from build123d import *

# Parameters (mm, degrees)
SKETCH1_R           = 4.5
BOSS_EXTRUDE1_DEPTH = 8
SKETCH2_R           = 4
BOSS_EXTRUDE2_DEPTH = 3
SKETCH3_R           = 2
CUT_EXTRUDE1_DEPTH  = 5
BOSS_EXTRUDE3_DEPTH = 8
SKETCH5_W           = 7
SKETCH5_H           = 20
BOSS_EXTRUDE4_DEPTH = 12
FILLET1_START       = -13.395559342
FILLET1_DEPTH       = 7
FILLET1_2_DEPTH     = 7
SKETCH6_W           = 7
SKETCH6_H           = 8
CUT_EXTRUDE2_DEPTH  = 8
FILLET2_R           = 3
SKETCH7_R           = 1.75
CUT_EXTRUDE3_DEPTH  = 57.724097483


with BuildPart() as part:
    # Sketch1 → Boss-Extrude1 (new body)
    with BuildSketch(Plane(origin=(0, 0, 0), x_dir=(1, 0, 0), z_dir=(0, 1, 0))):
        with BuildLine():
            Line((0, 6), (11, 6))
            Line((11, 6), (11, -6))
            Line((11, -6), (0, -6))
            ThreePointArc((0, -6), (-6, 0), (0, 6))
        make_face()
        with Locations(Location((0, 0, 0), (0, 0, 270))):
            Circle(SKETCH1_R, mode=Mode.SUBTRACT)
    extrude(amount=BOSS_EXTRUDE1_DEPTH)

    # Sketch2 → Boss-Extrude2 (add)
    with BuildSketch(Plane(origin=(11, 0, 0), x_dir=(0, 0, -1), z_dir=(1, 0, 0))):
        with Locations(Location((0, 4, 0), (0, 0, 270))):
            Circle(SKETCH2_R)
    extrude(amount=BOSS_EXTRUDE2_DEPTH)

    # Sketch3 → Cut-Extrude1 (cut)
    with BuildSketch(Plane(origin=(14, 0, 0), x_dir=(0, 0, -1), z_dir=(1, 0, 0))):
        with Locations((0, 4)):
            Circle(SKETCH3_R)
    extrude(amount=-CUT_EXTRUDE1_DEPTH, mode=Mode.SUBTRACT)

    # Sketch4 → Boss-Extrude3 (add)
    with BuildSketch(Plane(origin=(0, 0, 0), x_dir=(1, 0, 0), z_dir=(0, 1, 0))):
        Polygon((0, -6), (0, -9.124355653), (-13.395559342, -32.326145029), (-13.395559342, -39.201789376), (-6.395559342, -39.201789376), (-6.395559342, -34.201789376), (7, -11), (7, -6), align=None)
    extrude(amount=BOSS_EXTRUDE3_DEPTH)

    # Sketch5 → Boss-Extrude4 (add)
    with BuildSketch(Plane.XY.offset(39.201789376)):
        with Locations((-9.895559342, 4)):
            Rectangle(SKETCH5_W, SKETCH5_H)
    extrude(amount=BOSS_EXTRUDE4_DEPTH)

    # Fillet1: read off the stored shape, not the designer's step
    # Fillet1 outline → Fillet1 (cut)
    with BuildSketch(Plane.YZ.offset(FILLET1_START)):
        with BuildLine():
            Line((-6, 39.201789376), (-3, 39.201789376))
            ThreePointArc((-3, 39.201789376), (-5.121320344, 40.080469032), (-6, 42.201789376))
            Line((-6, 42.201789376), (-6, 39.201789376))
        make_face()
        with BuildLine():
            ThreePointArc((14, 42.201789376), (13.121320344, 40.080469032), (11, 39.201789376))
            Line((11, 39.201789376), (14, 39.201789376))
            Line((14, 39.201789376), (14, 42.201789376))
        make_face()
    extrude(amount=FILLET1_DEPTH, mode=Mode.SUBTRACT)

    # Fillet1 2 outline → Fillet1 2 (add)
    with BuildSketch(Plane.YZ.offset(FILLET1_START)):
        with BuildLine():
            ThreePointArc((-3, 39.201789376), (-0.878679657, 38.32310972), (0, 36.201789376))
            Line((0, 36.201789376), (0, 39.201789376))
            Line((0, 39.201789376), (-3, 39.201789376))
        make_face()
        with BuildLine():
            ThreePointArc((8, 36.201789376), (8.878679656, 38.32310972), (11, 39.201789376))
            Line((11, 39.201789376), (8, 39.201789376))
            Line((8, 39.201789376), (8, 36.201789376))
        make_face()
    extrude(amount=FILLET1_2_DEPTH)

    # Sketch6 → Cut-Extrude2 (cut)
    with BuildSketch(Plane.XY.offset(51.201789376)):
        with Locations((-9.895559342, 4)):
            Rectangle(SKETCH6_W, SKETCH6_H)
    extrude(amount=-CUT_EXTRUDE2_DEPTH, mode=Mode.SUBTRACT)

    # Fillet2
    fillet2_edges = [part.edges().sort_by_distance(p)[0] for p in [
        (-6.395559342, -3, 51.201789376),
        (-13.395559342, 11, 51.201789376),
        (-6.395559342, 11, 51.201789376),
        (-13.395559342, -3, 51.201789376),
    ]]
    fillet(fillet2_edges, radius=FILLET2_R)

    # Sketch7 → Cut-Extrude3 (cut, through all)
    with BuildSketch(Plane(origin=(0, 14, 0), x_dir=(1, 0, 0), z_dir=(0, 1, 0))):
        with Locations(Location((-9.895559342, -47.201789376, 0), (0, 0, 180))):
            Circle(SKETCH7_R)
    extrude(amount=-CUT_EXTRUDE3_DEPTH, mode=Mode.SUBTRACT)


solid = part.part
Read the model definition and answer for the solid it produces. Units are mm, in the model's axes. A direction names the side the tool comes from. Give positions to 0.01 mm unless a question says otherwise; leave off trailing zeros. Loops run counter-clockwise (first coordinate to the right, second up) from the corner with the lowest first, then second, coordinate; pieces in that order, holes last. Notation, with made-up numbers: (76, 46) -> (94, 46) arc R27 ccw to (94, 76) -> close; hole circle Ø9 at (-27.5, 52.5). An arc over 180 degrees is marked (long way). Use a Markdown table: item, result.
Q1. Section B-B, the plane x = 9.75 is taken. Determine the outline of the cut face in (y, z).
Solved:
| item | result |
|---|---|
| outline | (0, -6) -> (8, -6) -> (8, 6) -> (0, 6) -> close; hole circle Ø4 at (4, 0) |
Q2. Find the intervals of material crossed by line 1 along Z through (x, y) = (-1, 2.5); line 2 along Y through (x, z) = (-6.5, 45); line 3 along Y through (x, z) = (-4.5, 1.5), in increasing order.
Solved:
| item | result |
|---|---|
| line 1 | z = -5.92 to -4.39, 4.39 to 5.92, 10.86 to 24.86 |
| line 2 | y = -6 to 0, 8 to 14 |
| line 3 | y = 0 to 8 |
Q3. A tool of negligible diameter and unlimited length cuts with its end or side. For faces 5 (the face through (-6.396, 4, 41)), 6 (the face through (-12, 8, 46)), 7 (the face through (11, 3.9, -4.4)), 8 (the face through (0, 4, 8)), from which of +Z, -Z, +X, -X, +Y, -Y can it reach the whole face along a straight path? Write none if from no direction.
Solved:
| item | result |
|---|---|
| face 5 | +Z, +X, +Y, -Y |
| face 6 | +Z, +X, -X |
| face 7 | -Z, +X |
| face 8 | -X, +Y, -Y |
Q4. Section A-A, the plane y = 4 is taken. Determine the outline of the cut face in (x, z).
Solved:
| item | result |
|---|---|
| outline | (-13.4, 32.33) -> (0, 9.12) -> (0, 6) arc R6 ccw to (0, -6) -> (11, -6) -> (11, -4) -> (14, -4) -> (14, -2) -> (9, -2) -> (9, 2) -> (14, 2) -> (14, 4) -> (11, 4) -> (11, 6) -> (7, 6) -> (7, 11) -> (-6.4, 34.2) -> (-6.4, 43.2) -> (-13.4, 43.2) -> close; hole circle Ø9 at (0, 0) |
Q5. Determine the mould class of faces 1 (the face through (-12.54, -2.96, 50.3)), 2 (the face through (9, 4, 6)), 3 (the face through (11, 3.9, 4.3)), 4 (the face through (1.352, 3.944, 4.292)) for opening direction X: pulls with the +X half, pulls with the -X half, needs draft (parallel to the pull), parting line crosses it, or undercut.
Solved:
| item | result |
|---|---|
| face 1 | pulls with the -X half |
| face 2 | needs draft |
| face 3 | pulls with the +X half |
| face 4 | undercut |
Q6. Section C-C, the plane x = -3 is taken. Determine the outline of the cut face in (y, z), then the cut area to 3 significant figures.
Solved:
| item | result |
|---|---|
| outline | (0, -5.2) -> (8, -5.2) -> (8, -3.35) -> (0, -3.35) -> close; (0, 3.35) -> (8, 3.35) -> (8, 5.2) -> (0, 5.2) -> close; (0, 14.32) -> (8, 14.32) -> (8, 28.32) -> (0, 28.32) -> close |
| area | 141 mm^2 |
Q7. Each of these flat-tipped pins is pushed along its axis until it touches: pin 1 (1.5 mm diameter, centred on x = 10.5, y = 9, fed in from -Z); pin 2 (12 mm diameter, centred on x = -4, z = 6, fed in from -Y); pin 3 (4.5 mm diameter, centred on x = 9.5, y = 5, fed in from +Z); pin 4 (10 mm diameter, centred on y = 8, z = 3.5, fed in from -X). Where does it stop, or does it pass through?
Solved:
| item | result |
|---|---|
| pin 1 | passes through |
| pin 2 | stops at y = 0 |
| pin 3 | stops at z = 6 |
| pin 4 | stops at x = -6 |
Q8. Section D-D, the plane y = -1.5 is taken. Determine the outline of the cut face in (x, z), then the cut area to 3 significant figures.
Solved:
| item | result |
|---|---|
| outline | (-13.4, 38.8) -> (-6.4, 38.8) -> (-6.4, 48.2) arc R3 ccw to (-9.4, 51.2) -> (-10.4, 51.2) arc R3 ccw to (-13.4, 48.2) -> close; hole circle Ø3.5 at (-9.9, 47.2) |
| area | 73.3 mm^2 |
